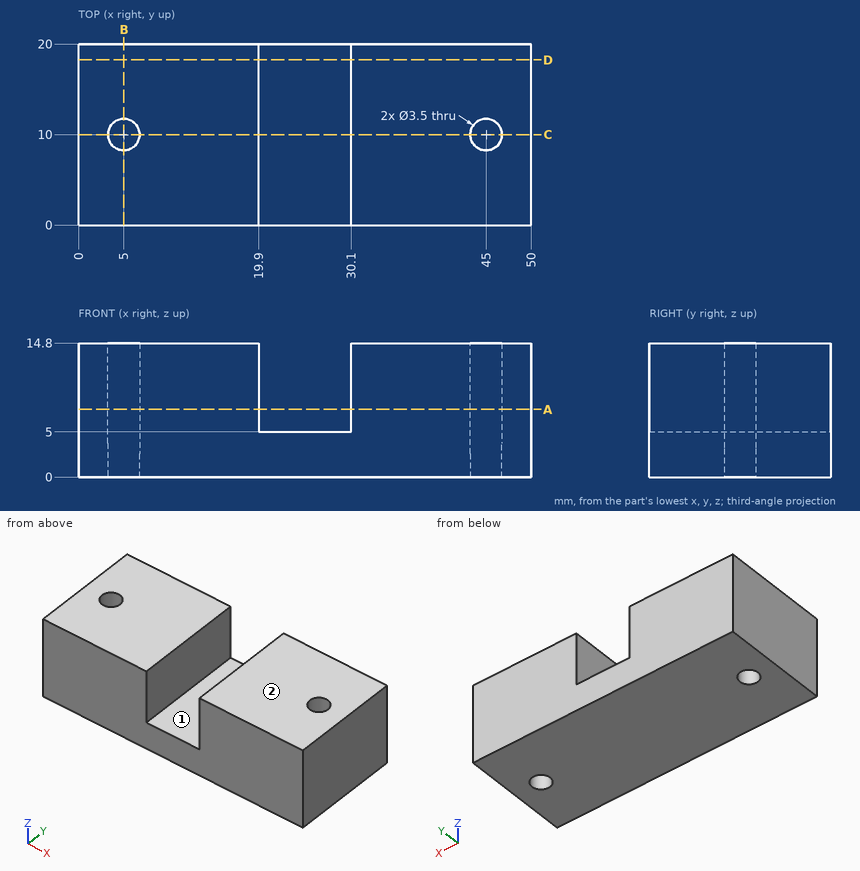
Source: three-view drawing plus pictorial views. Frame: mm from the lowest corner of the part. A direction names the side the tool comes from. Round coordinates to 2 decimals unless told otherwise and drop trailing zeros. Write each loop counter-clockwise with the first axis right and the second up, starting at its lowest first coordinate (ties: lowest second). Pieces come first, ordered by that corner, then holes. Notation, with made-up numbers: M 52,76 L 103,76 A22 cw 103,110 Z; hole C 31,6.5 d2. An arc over 180 degrees is marked long. Write each question's results on one line, items separated by ' | '.
Q1. Section query D-D (y = 18.25). Return loops of the section in (x, z), and give its area (3 significant figures).
Results:
outline: M 0,0 L 50,0 L 50,14.8 L 30.1,14.8 L 30.1,5 L 19.9,5 L 19.9,14.8 L 0,14.8 Z | area: 640 mm^2
Q2. Line query: line 1 along X through (y, z) = (16, 13.75); line 2 along Y through (x, z) = (45, 11.75); line 3 along X through (y, z) = (10.75, 10). Output: solid intervals per line, ascending.
Results:
line 1: x = 0 to 19.9, 30.1 to 50 | line 2: y = 0 to 8.25, 11.75 to 20 | line 3: x = 0 to 3.42, 6.58 to 19.9, 30.1 to 43.42, 46.58 to 50
Q3. Access query for the marked faces 1 and 2. Directions: +Z, -Z, +X, -X, +Y, -Y. A direction counts if a zero-diameter tool reaches every point of the face in a straight line with its end or side. Return the directions, or none.
Results:
face 1: +Z, +Y, -Y | face 2: +Z, +X, -X, +Y, -Y
Q4. Section query C-C (y = 10). Return loops of the section in (x, z), and give its area (3 significant figures).
Results:
outline: M 0,0 L 3.25,0 L 3.25,14.8 L 0,14.8 Z; M 6.75,0 L 43.25,0 L 43.25,14.8 L 30.1,14.8 L 30.1,5 L 19.9,5 L 19.9,14.8 L 6.75,14.8 Z; M 46.75,0 L 50,0 L 50,14.8 L 46.75,14.8 Z | area: 536 mm^2
Q5. Section query B-B (x = 5). Return loops of the section in (y, z).
Results:
outline: M 0,0 L 8.25,0 L 8.25,14.8 L 0,14.8 Z; M 11.75,0 L 20,0 L 20,14.8 L 11.75,14.8 Z
Q6. Pin query (flat end, axial travel): P1, Ø5, axis at x = 23.5, y = 9, coming from the +Z side. Return the tip coordinate at first contact, or that it passes through.
Results:
P1: stops at z = 5
Q7. Section query A-A (z = 7.5). Return loops of the section in (x, y).
Results:
outline: M 0,0 L 19.9,0 L 19.9,20 L 0,20 Z; M 30.1,0 L 50,0 L 50,20 L 30.1,20 Z; hole C 5,10 d3.5; hole C 45,10 d3.5
